```python
from build123d import *

# Parameters (mm, degrees)
SKETCH2_R           = 25.25
SKETCH2_R_2         = 20.25
BOSS_EXTRUDE1_DEPTH = 10
SKETCH3_R           = 30.4
SKETCH3_R_2         = 19.25
BOSS_EXTRUDE2_DEPTH = 30
SKETCH4_R           = 25.5
CUT_EXTRUDE1_DEPTH  = 29
CHAMFER2_SIZE       = 0.5


with BuildPart() as part:
    # Sketch2 → Boss-Extrude1 (new body)
    with BuildSketch(Plane.XY):
        Circle(SKETCH2_R)
        Circle(SKETCH2_R_2, mode=Mode.SUBTRACT)
    extrude(amount=BOSS_EXTRUDE1_DEPTH)

    # Sketch3 → Boss-Extrude2 (add)
    with BuildSketch(Plane(origin=(0, 0, 0), x_dir=(-1, 0, 0), z_dir=(0, 0, -1))):
        Circle(SKETCH3_R)
        Circle(SKETCH3_R_2, mode=Mode.SUBTRACT)
    extrude(amount=BOSS_EXTRUDE2_DEPTH)

    # Sketch4 → Cut-Extrude1 (cut)
    with BuildSketch(Plane(origin=(0, 0, -30), x_dir=(-1, 0, 0), z_dir=(0, 0, -1))):
        Circle(SKETCH4_R)
    extrude(amount=-CUT_EXTRUDE1_DEPTH, mode=Mode.SUBTRACT)

    # Chamfer2
    chamfer2_edges = [part.edges().sort_by_distance(p)[0] for p in [
        (19.25, 0, 0),
    ]]
    chamfer(chamfer2_edges, length=CHAMFER2_SIZE)


solid = part.part
```
Can you work these out from the model? Positions are in its coordinate system, mm. A direction names the side the tool comes from. Round coordinates to 2 decimals unless told otherwise and drop trailing zeros. Loops run counter-clockwise (first coordinate to the right, second up) from the corner with the lowest first, then second, coordinate; pieces in that order, holes last. Notation, with made-up numbers: (70, 34) -> (84, 34) arc R4 cw to (84, 39) -> close; hole circle Ø7 at (76, 48.5). An arc over 180 degrees is marked (long way). Answer in a Markdown table with one row per item.
Item 1: Suppose I cut it at D-D, the plane z = -5. List the corners of the cut face in (x, y) for me.
Answer block:
| item | result |
|---|---|
| outline | circle Ø60.8 at (0, 0); hole circle Ø51 at (0, 0) |
Item 2: Suppose I cut it at C-C, the plane z = 2. List the corners of the cut face in (x, y) for me.
Answer block:
| item | result |
|---|---|
| outline | circle Ø50.5 at (0, 0); hole circle Ø40.5 at (0, 0) |
Item 3: Will these pins go through, and if not, where does the flat tip stop? P1, Ø1, axis at y = 10.5, z = -25.5, coming from the +X side; P2, Ø3, axis at y = 8.5, z = 0.5, coming from the -X side; P3, Ø1, axis at x = 4.5, z = -19.5, coming from the +Y side.
Answer block:
| item | result |
|---|---|
| P1 | x = 28.71 |
| P2 | x = -29.56 |
| P3 | y = 30.14 |
Item 4: On a 3-axis mill with a long thin cutter (end or side, diameter ignored), from which of +Z, -Z, +X, -X, +Y, -Y can I reach the whole of each face in a straight line? I mean faces 4 (the cylindrical face through (15.28, -11.71, -0.75)), 5 (the flat face through (-4.41, -19.41, 0)), 6 (the cylindrical face through (5.5, -24.9, -15.7)). Say none if no direction works.
Answer block:
| item | result |
|---|---|
| face 4 | +Z, -Z |
| face 5 | +Z |
| face 6 | -Z |
Item 5: If I drill on probe 1 along Y at (x, z) = (0, -0.55); probe 2 along X at (y, z) = (-0.5, 3.5); probe 3 along Y at (x, z) = (0, 6.75), over which ranges is the centre line in solid material (lowest first)?
Answer block:
| item | result |
|---|---|
| probe 1 | -30.4 to -19.25, 19.25 to 30.4 |
| probe 2 | -25.25 to -20.24, 20.24 to 25.25 |
| probe 3 | -25.25 to -20.25, 20.25 to 25.25 |
Item 6: We'd pull the mould along X, two halves only. Please class faces 1 (the flat face through (-19, 8, 10)), 2 (the cylindrical face through (11, 17, 5)), 3 (the cylindrical face through (30.37, 1.34, -14.79)): released by +X, released by -X, zero draft, split by the parting line, or undercut.
Answer block:
| item | result |
|---|---|
| face 1 | zero draft |
| face 2 | undercut |
| face 3 | split by the parting line |
Item 7: Suppose I cut it at A-A, the plane x = 0. List the corners of the cut face in (y, z) for me.
Answer block:
| item | result |
|---|---|
| outline | (-30.4, -30) -> (-25.5, -30) -> (-25.5, -1) -> (-19.25, -1) -> (-19.25, -0.5) -> (-19.75, 0) -> (-20.25, 0) -> (-20.25, 10) -> (-25.25, 10) -> (-25.25, 0) -> (-30.4, 0) -> close; (19.25, -1) -> (25.5, -1) -> (25.5, -30) -> (30.4, -30) -> (30.4, 0) -> (25.25, 0) -> (25.25, 10) -> (20.25, 10) -> (20.25, 0) -> (19.75, 0) -> (19.25, -0.5) -> close |
